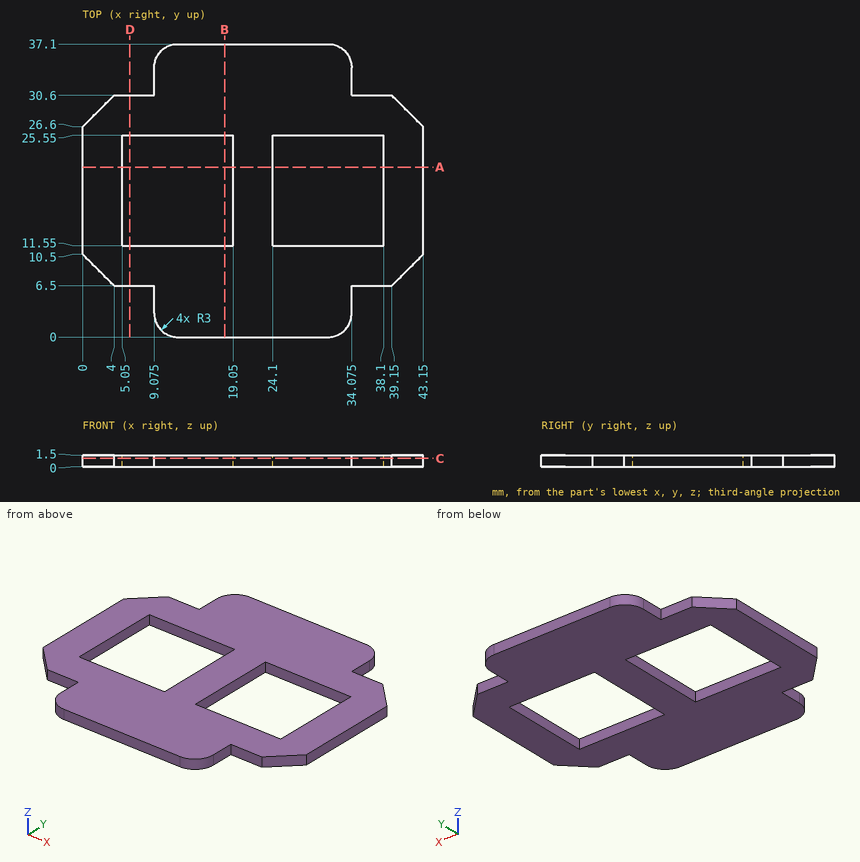
For this review, use the dimensioned drawing (mm, ordinates from the lowest corner) and the shaded views. Coordinates: 2 decimals unless noted, no trailing zeros. Loops run counter-clockwise (first coordinate to the right, second up) from the corner with the lowest first, then second, coordinate; pieces in that order, holes last.
1. Insertion check: P1, Ø0.8, axis at x = 36, z = 1, coming from the -Y side; P2, Ø6, axis at x = 30, y = 19, coming from the -Z side; P3, Ø0.8, axis at y = 5, z = 1, coming from the -X side (3 decimals). Each pin has a flat end and moves straight along its axis. Give the tip position at first contact, or say it passes through.
2. Add section B-B, the plane x = 18. Give the boundary of the cut face in (y, z), then the cut area to 4 significant figures.
3. For line 1 (X direction, y = 20, z = 0.8); line 2 (Y direction, x = 29.5, z = 0.2); line 3 (Y direction, x = 37, z = 1.3), list the stretches that pass through material, from the lowest coordinate up.
4. Add section A-A, the plane y = 21.5. Give the boundary of the cut face in (x, z), then the cut area to 3 significant figures.
5. Add section D-D, the plane x = 6. Give the boundary of the cut face in (y, z), then the cut area to 4 significant figures.
6. Add section C-C, the plane z = 1.1. Give the boundary of the cut face in (x, y) (3 decimals).
Result:
1. P1: stops at y = 6.5
1. P2: passes through
1. P3: stops at x = 9.075
2. outline: (0, 0) - (11.55, 0) - (11.55, 1.5) - (0, 1.5) - close; (25.55, 0) - (37.1, 0) - (37.1, 1.5) - (25.55, 1.5) - close
2. area: 34.65 mm2
3. line 1: x = 0 to 5.05, 19.05 to 24.1, 38.1 to 43.15
3. line 2: y = 0 to 11.55, 25.55 to 37.1
3. line 3: y = 6.5 to 11.55, 25.55 to 30.6
4. outline: (0, 0) - (5.05, 0) - (5.05, 1.5) - (0, 1.5) - close; (19.05, 0) - (24.1, 0) - (24.1, 1.5) - (19.05, 1.5) - close; (38.1, 0) - (43.15, 0) - (43.15, 1.5) - (38.1, 1.5) - close
4. area: 22.7 mm2
5. outline: (6.5, 0) - (11.55, 0) - (11.55, 1.5) - (6.5, 1.5) - close; (25.55, 0) - (30.6, 0) - (30.6, 1.5) - (25.55, 1.5) - close
5. area: 15.15 mm2
6. outline: (0, 10.5) - (4, 6.5) - (9.075, 6.5) - (9.075, 3) arc R3 ccw to (12.075, 0) - (31.075, 0) arc R3 ccw to (34.075, 3) - (34.075, 6.5) - (39.15, 6.5) - (43.15, 10.5) - (43.15, 26.6) - (39.15, 30.6) - (34.075, 30.6) - (34.075, 34.1) arc R3 ccw to (31.075, 37.1) - (12.075, 37.1) arc R3 ccw to (9.075, 34.1) - (9.075, 30.6) - (4, 30.6) - (0, 26.6) - close; hole (5.05, 11.55) - (19.05, 11.55) - (19.05, 25.55) - (5.05, 25.55) - close; hole (24.1, 11.55) - (38.1, 11.55) - (38.1, 25.55) - (24.1, 25.55) - close
